CAD build for the part. Positions are in the model's coordinates, mm. A direction names the side the tool comes from. Round coordinates to 2 decimals unless told otherwise and drop trailing zeros. Order: outer loops, then holes, each group sorted by start corner. A loop starts at its lowest first (then second) coordinate and runs counter-clockwise, first axis right, second up. Notation, with made-up numbers: M 29,44 L 68,44 A12 ccw 68,53 Z; hole C 51,-22 d8. An arc over 180 degrees is marked long. Answer as a JSON object with one key per item and string values. Group by question number.
```python
from build123d import *

# Parameters (mm, degrees)
F0_W          = 654.05
F0_H          = 2413
F0_W_2        = 584.2
F0_H_2        = 317.5
F0_H_3        = 1625.6
F1_DEPTH      = 22.225
F1_DEPTH_BACK = 22.225
F2_W          = 1248.5843106929
F2_H          = 271.0993243682
F2_H_2        = 504.0157202398
F3_DEPTH      = 22.226
F3_DEPTH_BACK = 22.226


# Not quite as in the source:
# - a length typed as a fraction of an inch, garbled in the dataset ("3 / 203.2 mm" for 3/8 in), is restored


with BuildPart() as f1:
    # F0 (on Front) → F1 (new body, two sides)
    with BuildSketch(Plane.XZ) as f1_sk:
        Rectangle(F0_W, F0_H)
        with Locations((0, -822.325)):
            Rectangle(F0_W_2, F0_H_2, mode=Mode.SUBTRACT)
        with Locations((0, 263.525)):
            Rectangle(F0_W_2, F0_H_3, mode=Mode.SUBTRACT)
    extrude(amount=F1_DEPTH)
    extrude(f1_sk.sketch, amount=-F1_DEPTH_BACK)

    # F2 (on Front) → F3 (cut, two sides)
    with BuildSketch(Plane.XZ) as f3_sk:
        with Locations((62.8663003445, 1342.0496621841)):
            Rectangle(F2_W, F2_H)
        with Locations((62.8663003445, -1382.3078601199)):
            Rectangle(F2_W, F2_H_2)
    extrude(amount=-F3_DEPTH, mode=Mode.SUBTRACT)
    extrude(f3_sk.sketch, amount=F3_DEPTH_BACK, mode=Mode.SUBTRACT)


solid = f1.part
```
Item 1: Drill centre lines: line 1 (Z direction, x = 277, y = 9) (3 decimals); line 2 (X direction, y = -12.5, z = -920.5) (3 decimals). Where is each one in solid material? Low to high. Write a range as [from, to].
Item 2: Cut at A-A, the plane z = 908. Give the cut face in (x, y) (3 decimals).
Item 3: 3-axis set-ups, long thin cutter, end or side, ignore diameter. For faces 1 (the face through (-5, 0, 1206.5)), 2 (the face through (292.1, 0, 252)): which of +Z, -Z, +X, -X, +Y, -Y reach the whole face in a straight line?
Item 4: Cut at C-C, the plane x = 115. Give the cut face in (y, z) (3 decimals), and give its area (3 significant figures).
Item 5: Cut at B-B, the plane y = 11.5. Give the cut face in (x, z) (3 decimals), and give its area (3 significant figures).
Item 6: Two-plate mould, pull along X, no slides. Class faces 3 (the face through (-316, -22.225, -216)), 4 (the face through (-4, 0, -981.075)), 5 (the face through (-327.025, 0, 22)): +X half, -X half, draft (parallel to the pull), parting line (faces both ways), or undercut.
Response values:
{
 "1": {"line 1": "[-1130.3, -981.075], [-663.575, -549.275], [1076.325, 1206.5]", "line 2": "[-327.025, -292.1], [292.1, 327.025]"},
 "2": {"outline": "M -327.025,-22.225 L -292.1,-22.225 L -292.1,22.225 L -327.025,22.225 Z; M 292.1,-22.225 L 327.025,-22.225 L 327.025,22.225 L 292.1,22.225 Z"},
 "3": {"face 1": "+Z, +X, -X, +Y, -Y", "face 2": "+Y, -Y"},
 "4": {"outline": "M -22.225,-1130.3 L 22.225,-1130.3 L 22.225,-981.075 L -22.225,-981.075 Z; M -22.225,-663.575 L 22.225,-663.575 L 22.225,-549.275 L -22.225,-549.275 Z; M -22.225,1076.325 L 22.225,1076.325 L 22.225,1206.5 L -22.225,1206.5 Z", "area": "17,500 mm^2"},
 "5": {"outline": "M -327.025,-1130.3 L 327.025,-1130.3 L 327.025,1206.5 L -327.025,1206.5 Z; hole M -292.1,-981.075 L 292.1,-981.075 L 292.1,-663.575 L -292.1,-663.575 Z; hole M -292.1,-549.275 L 292.1,-549.275 L 292.1,1076.325 L -292.1,1076.325 Z", "area": "393,000 mm^2"},
 "6": {"face 3": "draft", "face 4": "undercut", "face 5": "-X half"}
}
